```python
from build123d import *

# Parameters (mm, degrees)
RESSALTO_EXTRUS_O1_DEPTH = 18
CORTE_EXTRUS_O1_DEPTH    = 2
CORTE_EXTRUS_O2_DEPTH    = 31
ESBO_O4_R                = 2.5
ESBO_O4_R_2              = 1.5
RESSALTO_EXTRUS_O2_DEPTH = 5
ESBO_O5_R                = 2.5
ESBO_O5_R_2              = 1.5
RESSALTO_EXTRUS_O3_DEPTH = 31


with BuildPart() as part:
    # Esboço1 → Ressalto-extrusão1 (new, symmetric)
    with BuildSketch(Plane.XY):
        with BuildLine():
            Line((-70, -48.5), (70, -48.5))
            ThreePointArc((70, -48.5), (72.828427125, -47.328427125), (74, -44.5))
            Line((74, -44.5), (74, 44.5))
            ThreePointArc((74, 44.5), (72.828427125, 47.328427125), (70, 48.5))
            Line((70, 48.5), (-70, 48.5))
            ThreePointArc((-70, 48.5), (-72.828427125, 47.328427125), (-74, 44.5))
            Line((-74, 44.5), (-74, -44.5))
            ThreePointArc((-74, -44.5), (-72.828427125, -47.328427125), (-70, -48.5))
        make_face()
    extrude(amount=RESSALTO_EXTRUS_O1_DEPTH, both=True)

    # Esboço2 → Corte-extrusão1 (cut)
    with BuildSketch(Plane.XY.offset(18)):
        with BuildLine():
            Line((-68, -47), (68, -47))
            ThreePointArc((68, -47), (70.828427125, -45.828427125), (72, -43))
            Line((72, -43), (72, 43))
            ThreePointArc((72, 43), (70.828427125, 45.828427125), (68, 47))
            Line((68, 47), (-68, 47))
            ThreePointArc((-68, 47), (-70.828427125, 45.828427125), (-72, 43))
            Line((-72, 43), (-72, -43))
            ThreePointArc((-72, -43), (-70.828427125, -45.828427125), (-68, -47))
        make_face()
    extrude(amount=-CORTE_EXTRUS_O1_DEPTH, mode=Mode.SUBTRACT)

    # Esboço3 → Corte-extrusão2 (cut)
    with BuildSketch(Plane.XY.offset(16)):
        with BuildLine():
            Line((-67, -46), (67, -46))
            ThreePointArc((67, -46), (69.828427125, -44.828427125), (71, -42))
            Line((71, -42), (71, 42))
            ThreePointArc((71, 42), (69.828427125, 44.828427125), (67, 46))
            Line((67, 46), (-67, 46))
            ThreePointArc((-67, 46), (-69.828427125, 44.828427125), (-71, 42))
            Line((-71, 42), (-71, -42))
            ThreePointArc((-71, -42), (-69.828427125, -44.828427125), (-67, -46))
        make_face()
    extrude(amount=-CORTE_EXTRUS_O2_DEPTH, mode=Mode.SUBTRACT)

    # Esboço4 → Ressalto-extrusão2 (add)
    # profile 1 of 8: a face of its own
    with BuildSketch(Plane.XY.offset(-15)):
        with Locations(Location((-28, 29.5, 0), (0, 0, 180))):
            Circle(ESBO_O4_R)
        with Locations((-28, 29.5)):
            Circle(ESBO_O4_R_2, mode=Mode.SUBTRACT)
    # profile 2 of 8: a face of its own
    with BuildSketch(Plane.XY.offset(-15)):
        with Locations(Location((28, 29.5, 0), (0, 0, 180))):
            Circle(ESBO_O4_R)
        with Locations((28, 29.5)):
            Circle(ESBO_O4_R_2, mode=Mode.SUBTRACT)
    # profile 3 of 8: a face of its own
    with BuildSketch(Plane.XY.offset(-15)):
        with Locations(Location((28, -29.5, 0), (0, 0, 180))):
            Circle(ESBO_O4_R)
        with Locations((28, -29.5)):
            Circle(ESBO_O4_R_2, mode=Mode.SUBTRACT)
    # profile 4 of 8: a face of its own
    with BuildSketch(Plane.XY.offset(-15)):
        with Locations(Location((-28, -29.5, 0), (0, 0, 180))):
            Circle(ESBO_O4_R)
        with Locations((-28, -29.5)):
            Circle(ESBO_O4_R_2, mode=Mode.SUBTRACT)
    # profile 5 of 8: a face of its own
    with BuildSketch(Plane.XY.offset(-15)):
        with Locations(Location((-48, 22, 0), (0, 0, 180))):
            Circle(ESBO_O4_R)
        with Locations((-48, 22)):
            Circle(ESBO_O4_R_2, mode=Mode.SUBTRACT)
    # profile 6 of 8: a face of its own
    with BuildSketch(Plane.XY.offset(-15)):
        with Locations(Location((-48, -22, 0), (0, 0, 180))):
            Circle(ESBO_O4_R)
        with Locations((-48, -22)):
            Circle(ESBO_O4_R_2, mode=Mode.SUBTRACT)
    # profile 7 of 8: a face of its own
    with BuildSketch(Plane.XY.offset(-15)):
        with Locations(Location((48, -22, 0), (0, 0, 180))):
            Circle(ESBO_O4_R)
        with Locations((48, -22)):
            Circle(ESBO_O4_R_2, mode=Mode.SUBTRACT)
    # profile 8 of 8: a face of its own
    with BuildSketch(Plane.XY.offset(-15)):
        with Locations(Location((48, 22, 0), (0, 0, 180))):
            Circle(ESBO_O4_R)
        with Locations((48, 22)):
            Circle(ESBO_O4_R_2, mode=Mode.SUBTRACT)
    extrude(amount=RESSALTO_EXTRUS_O2_DEPTH)

    # Esboço5 → Ressalto-extrusão3 (add)
    # profile 1 of 4: a face of its own
    with BuildSketch(Plane.XY.offset(-15)):
        with Locations(Location((-67, -42.5, 0), (0, 0, 180))):
            Circle(ESBO_O5_R)
        with Locations(Location((-67, -42.5, 0), (0, 0, 180))):
            Circle(ESBO_O5_R_2, mode=Mode.SUBTRACT)
    # profile 2 of 4: a face of its own
    with BuildSketch(Plane.XY.offset(-15)):
        with Locations(Location((67, -42.5, 0), (0, 0, 180))):
            Circle(ESBO_O5_R)
        with Locations(Location((67, -42.5, 0), (0, 0, 180))):
            Circle(ESBO_O5_R_2, mode=Mode.SUBTRACT)
    # profile 3 of 4: a face of its own
    with BuildSketch(Plane.XY.offset(-15)):
        with Locations(Location((67, 42.5, 0), (0, 0, 180))):
            Circle(ESBO_O5_R)
        with Locations(Location((67, 42.5, 0), (0, 0, 180))):
            Circle(ESBO_O5_R_2, mode=Mode.SUBTRACT)
    # profile 4 of 4: a face of its own
    with BuildSketch(Plane.XY.offset(-15)):
        with Locations(Location((-67, 42.5, 0), (0, 0, 180))):
            Circle(ESBO_O5_R)
        with Locations(Location((-67, 42.5, 0), (0, 0, 180))):
            Circle(ESBO_O5_R_2, mode=Mode.SUBTRACT)
    extrude(amount=RESSALTO_EXTRUS_O3_DEPTH)


solid = part.part
```
Source: CAD feature listing. Evaluate the final solid. Frame: model axes, mm. Round coordinates to 2 decimals unless told otherwise and drop trailing zeros. Loops run counter-clockwise (first coordinate to the right, second up) from the corner with the lowest first, then second, coordinate; pieces in that order, holes last. Notation, with made-up numbers: M 56.25,37.25 L 60.25,37.25 A24 ccw 60.25,72.25 Z; hole C 79,1 d8. An arc over 180 degrees is marked long. Use a Markdown table: item, result. Add a question column.
1. Line query: line 1 (X direction, y = 42.5, z = 6.5); line 2 (Y direction, x = 67, z = 0); line 3 (Y direction, x = 28, z = -11.2). Output: solid intervals per line, ascending.
2. Mould query, pull axis X, two halves, no side actions, for faces 1 (the flat face through (-1, 1, -18)), 2 (the flat face through (48, 24, -10)), 3 (the flat face through (-74, 1, 0)). Classes: pulls with the +X half, pulls with the -X half, needs draft (parallel to the pull), parting line crosses it, or undercut.
3. Contact query for flat-ended pins moving along their axis: P1, Ø2.5, axis at x = -28, y = 29.5, coming from the +Z side; P2, Ø2.5, axis at x = 67.5, y = -43, coming from the +Z side; P3, Ø4, axis at x = -48.5, y = -21.5, coming from the +Z side. Output: stop coordinate, or through.
4. Section query C-C on y = -5.5. Return the cut outline in (x, z), then the cut area to 3 significant figures.
5. Section query D-D on x = -28. Return the cut outline in (y, z), then the cut area to 3 significant figures.
6. Section query A-A on z = -3. Give the number of separate pieces and of enclosed holes in the cut face, then the cut area to 3 significant figures.
7. Section query B-B on x = 36.5. Return the cut outline in (y, z), then the cut area to 3 significant figures.
Reported:
| question | item | result |
|---|---|---|
| 1 | line 1 | x = -74 to -70.97, -69.5 to -68.5, -65.5 to -64.5, 64.5 to 65.5, 68.5 to 69.5, 70.97 to 74 |
| 1 | line 2 | y = -48.5 to -46, -45 to -44, -41 to -40, 40 to 41, 44 to 45, 46 to 48.5 |
| 1 | line 3 | y = -48.5 to -46, -32 to -31, -28 to -27, 27 to 28, 31 to 32, 46 to 48.5 |
| 2 | face 1 | needs draft |
| 2 | face 2 | undercut |
| 2 | face 3 | pulls with the -X half |
| 3 | P1 | stops at z = -15 |
| 3 | P2 | stops at z = 16 |
| 3 | P3 | stops at z = -10 |
| 4 | outline | M -74,-18 L 74,-18 L 74,18 L 72,18 L 72,16 L 71,16 L 71,-15 L -71,-15 L -71,16 L -72,16 L -72,18 L -74,18 Z |
| 4 | area | 638 mm² |
| 5 | outline | M -48.5,-18 L 48.5,-18 L 48.5,18 L 47,18 L 47,16 L 46,16 L 46,-15 L 32,-15 L 32,-10 L 31,-10 L 31,-15 L 28,-15 L 28,-10 L 27,-10 L 27,-15 L -27,-15 L -27,-10 L -28,-10 L -28,-15 L -31,-15 L -31,-10 L -32,-10 L -32,-15 L -46,-15 L -46,16 L -47,16 L -47,18 L -48.5,18 Z |
| 5 | area | 472 mm² |
| 6 | separate pieces | 5 |
| 6 | enclosed holes | 5 |
| 6 | area | 1,340 mm² |
| 7 | outline | M -48.5,-18 L 48.5,-18 L 48.5,18 L 47,18 L 47,16 L 46,16 L 46,-15 L -46,-15 L -46,16 L -47,16 L -47,18 L -48.5,18 Z |
| 7 | area | 452 mm² |
